Input: part model. Units: mm. Frame: model coordinates. Face numbers are marked on the shaded views. Coordinates: 2 decimals unless noted, no trailing zeros. Write each loop counter-clockwise with the first axis right and the second up, starting at its lowest first coordinate (ties: lowest second). Pieces come first, ordered by that corner, then holes. Notation, with made-up numbers: (56, 76) - (97, 76) arc R24 cw to (97, 90) - close; hole circle Ø9 at (15, 42.25). An arc over 180 degrees is marked (long way). One line per question, with ' | ' between items. Start each with the question number.
1) First-contact query: P1, Ø5, axis at y = 22, z = 31.5, coming from the -X side; P2, Ø21.5, axis at x = -46.5, z = 9.5, coming from the -Y side; P3, Ø1.5, axis at x = 16.5, y = 1.5, coming from the -Z side; P4, Ø1.5, axis at x = -49.5, z = -12, coming from the -Y side (3 decimals). Flat tips, straight axial feed; report the tip coordinate or a pass-through.
2) Section query A-A on y = 24. Return loops of the section in (x, z), and give its area (3 significant figures).
3) Draft query along Z for the marked faces 1, 2 and 3. Return one class per face: released by +Z, released by -Z, zero draft, split by the parting line, or undercut.
4) Section query B-B on x = -40. Return loops of the section in (y, z).
5) Line query: line 1 (X direction, y = 29, z = -56); line 2 (Z direction, x = -6, y = 15.5); line 3 (X direction, y = 32, z = -28.5). Output: solid intervals per line, ascending.
6) Section query C-C on z = -38. Return loops of the section in (x, y), and give its area (3 significant figures).
```python
from build123d import *

# Parameters (mm, degrees)
F1_DEPTH = 47.752
F3_DEPTH = 125.8997323481
F5_W     = 28.5765696317
F5_H     = 79.3209560215
F6_DEPTH = 128.4397323481
F2_R     = 17.5244442396
F7_DEPTH = 3.0480007527


with BuildPart() as f1:
    # F0 (on Front) → F1 (new body, symmetric)
    with BuildSketch(Plane.XZ):
        with BuildLine():
            ThreePointArc((-61.5604854778, -17.279496366), (-64.1340028036, -53.9436351961), (-27.3913528199, -54.8708567219))
            Line((-27.3913528199, -54.8708567219), (16.5702632333, -19.2516883407))
            Line((16.5702632333, -19.2516883407), (14.5168037691, -16.992563549))
            Line((14.5168037691, -16.992563549), (-29.4344777615, -52.603358555))
            ThreePointArc((-29.4344777615, -52.603358555), (-61.8778750989, -51.8941968791), (-59.4991920915, -19.5303465483))
            Line((-59.4991920915, -19.5303465483), (-19.8167012668, 20.779631988))
            Line((-19.8167012668, 20.779631988), (-21.8700110068, 23.0385920597))
            Line((-21.8700110068, 23.0385920597), (-61.5604854778, -17.279496366))
        make_face()
        Polygon((14.5168037691, -16.992563549), (16.5702632333, -19.2516883407), (60.5318792866, 16.3674800405), (58.5385509124, 18.675325048), align=None)
        Polygon((17.8204634643, 63.3566804854), (-21.8700110068, 23.0385920597), (-19.8167012668, 20.779631988), (19.9267067724, 61.151491005), align=None)
        with BuildLine():
            Line((58.5385509124, 18.675325048), (60.5318792866, 16.3674800405))
            ThreePointArc((60.5318792866, 16.3674800405), (62.5637295367, 61.1204909666), (17.8204634643, 63.3566804854))
            Line((17.8204634643, 63.3566804854), (19.9267067724, 61.151491005))
            ThreePointArc((19.9267067724, 61.151491005), (60.3075985546, 59.0710562617), (58.5385509124, 18.675325048))
        make_face()
    extrude(amount=F1_DEPTH, both=True)

    # F2 (on face) → F3 (cut, through all)
    with BuildSketch(Plane(origin=(-22.624429106, 0, 22.272244566), x_dir=(0, -1, 0), z_dir=(-0.7126316385, 0, 0.7015384151))):
        Polygon((47.752, 2.3330547172), (47.752, 57.6517147172), (25.4, 2.3330547172), (25.4, -55.5009612218), (47.752, -55.5009612218), align=None)
    extrude(amount=-F3_DEPTH, mode=Mode.SUBTRACT)

    # F5 (on offset) → F6 (cut, through all)
    with BuildSketch(Plane(origin=(-24.4345134677, 0, 24.0541521404), x_dir=(0, -1, 0), z_dir=(-0.7126316385, 0, 0.7015384151))):
        with Locations((39.7184668109, -94.0875317901)):
            Rectangle(F5_W, F5_H)
    extrude(amount=-F6_DEPTH, mode=Mode.SUBTRACT)

    # F2 (on face) → F7 (cut, through all)
    with BuildSketch(Plane(origin=(-22.624429106, 0, 22.272244566), x_dir=(0, -1, 0), z_dir=(-0.7126316385, 0, 0.7015384151))):
        with Locations((0, 34.1488756239)):
            Circle(F2_R)
    extrude(amount=-F7_DEPTH, mode=Mode.SUBTRACT)


solid = f1.part
```
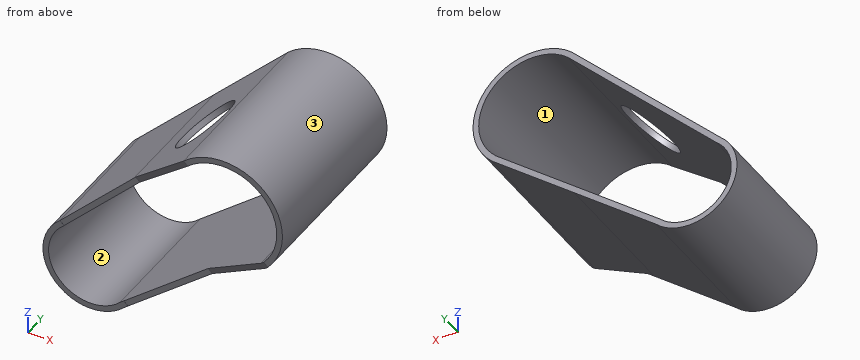
Answer key:
1) P1: x = -16 | P2: y = -25.4 | P3: z = -19.92 | P4: through
2) outline: (-61.56, -17.28) arc R25.43 ccw (long way) to (-27.39, -54.87) - (60.53, 16.37) arc R31.75 ccw to (17.82, 63.36) - close; hole (-59.5, -19.53) arc R22.38 ccw (long way) to (-29.43, -52.6) - (58.54, 18.68) arc R28.7 ccw to (19.93, 61.15) - close | area: 1,210 mm²
3) face 1: undercut | face 2: undercut | face 3: split by the parting line
4) outline: (-25.43, -61.7) - (47.75, -61.7) - (47.75, -58.58) - (-25.43, -58.58) - close; (-25.4, 0.28) - (47.75, 0.28) - (47.75, 4.62) - (-25.4, 4.62) - close
5) line 1: -62.04 to -56.88, -33.76 to -28.6 | line 2: -37.54 to -33.62, 34.81 to 39.16 | line 3: -69.34 to -66.08, 0.31 to 5.16
6) outline: (-70.72, -25.43) - (-67.67, -25.43) - (-67.67, 47.75) - (-70.72, 47.75) - close; (-11.41, -25.4) - (-6.57, -25.4) - (-6.57, 47.75) - (-11.41, 47.75) - close | area: 578 mm²
